Input: part model. Units: mm. Frame: model coordinates. A direction names the side the tool comes from. Give positions to 0.01 mm unless a question says otherwise; leave off trailing zeros. Loops run counter-clockwise (first coordinate to the right, second up) from the corner with the lowest first, then second, coordinate; pieces in that order, holes last. Notation, with made-up numbers: M 71,64 L 117,64 A25 cw 117,96 Z; hole C -17.5,18.5 d6. An arc over 180 degrees is marked long. Use CSV: the item, a comma, the result in double quotes. Start each with the question number.
from build123d import *

# Parameters (mm, degrees)
F1_DEPTH = 12.5
F2_R     = 6
F3_DEPTH = 20.001
F4_R     = 5
F5_R     = 12
F6_W     = 12
F6_H     = 90
F7_DEPTH = 20.001
F8_R     = 5.99999


# Not quite as in the source:
# - a fillet or chamfer is up to 0.001 mm smaller than in the source, because OpenCascade refuses the exact size


with BuildPart() as f1:
    # F0 (on Right) → F1 (new body, symmetric)
    with BuildSketch(Plane.YZ):
        Polygon((-6.25, 170), (-10, 170), (-10, -10), (10, -10), (10, 170), (6.25, 170), (6.25, 20), (-6.25, 20), align=None)
    extrude(amount=F1_DEPTH, both=True)

    # F2 (on face) → F3 (cut, through all)
    with BuildSketch(Plane.XZ.offset(10)):
        Circle(F2_R)
    extrude(amount=-F3_DEPTH, mode=Mode.SUBTRACT)

    # F4
    f4_edges = [f1.edges().sort_by_distance(p)[0] for p in [
        (12.5, 0, -10),
        (-12.5, 0, -10),
    ]]
    fillet(f4_edges, radius=F4_R)

    # F5
    f5_edges = [f1.edges().sort_by_distance(p)[0] for p in [
        (12.5, 0, 20),
        (-12.5, 0, 20),
    ]]
    fillet(f5_edges, radius=F5_R)

    # F6 (on face) → F7 (cut, through all)
    with BuildSketch(Plane.XZ.offset(10)):
        with Locations((0, 120)):
            Rectangle(F6_W, F6_H)
    extrude(amount=-F7_DEPTH, mode=Mode.SUBTRACT)

    # F8 (radius 6 in the source; OpenCascade refuses exactly that, so slightly less here)
    f8_edges = [f1.edges().sort_by_distance(p)[0] for p in [
        (-6, -8.125, 165),
        (6, -8.125, 165),
        (6, -8.125, 75),
        (-6, -8.125, 75),
        (-6, 8.125, 75),
        (6, 8.125, 75),
        (6, 8.125, 165),
        (-6, 8.125, 165),
    ]]
    fillet(f8_edges, radius=F8_R)


solid = f1.part
Item 1: Mould query, pull axis Y, two halves, no side actions, for faces 4 (the cylindrical face through (-4.196, 8.151, 76.711)), 5 (the flat face through (0, 10, 59)), 6 (the cylindrical face through (8.89, -0.09, 16.58)). Classes: +Y half, -Y half, draft (parallel to the pull), parting line (faces both ways), or undercut.
Item 2: Section A-A (z = 154.5). Output: boundary loops of the cut face in (x, y).
Item 3: Section B-B (z = 23.5). Output: boundary loops of the cut face in (x, y).
Item 4: Material intervals for line 1 (Y direction, x = 10, z = 45); line 2 (Z direction, x = 0, y = -3.5); line 3 (X direction, y = 2.25, z = 3), sorted ascending.
Item 5: Section D-D (z = 0). Output: boundary loops of the cut face in (x, y), then the cut area to 3 significant figures.
Item 6: First-contact query: pin 1 Ø9.5 at (x, z) = (0, 0) entering from +Y; pin 2 Ø3 at (x, y) = (9.5, 2) entering from +Z; pin 3 Ø0.8 at (x, y) = (0, -0.5) entering from +Z. Flat tips, straight axial feed; report the tip coordinate or a pass-through.
Item 7: Set-up query: faces 1 (the cylindrical face through (4.289, -8.099, 76.804)), 2 (the cylindrical face through (-9.08, -0.09, 16.39)), 3 (the cylindrical face through (11.07, 0.14, -8.5)). Return all of +Z, -Z, +X, -X, +Y, -Y with unobstructed straight access to the full face (end or side cutting, diameter ignored); none if empty.
Item 8: Section C-C (y = 3). Output: boundary loops of the cut face in (x, z), then the cut area to 3 significant figures.
Recorded:
1,face 4,"draft"
1,face 5,"+Y half"
1,face 6,"undercut"
2,outline,"M -12.5,-10 L -6,-10 L -6,-6.25 L -12.5,-6.25 Z; M -12.5,6.25 L -6,6.25 L -6,10 L -12.5,10 Z; M 6,-10 L 12.5,-10 L 12.5,-6.25 L 6,-6.25 Z; M 6,6.25 L 12.5,6.25 L 12.5,10 L 6,10 Z"
3,outline,"M -12.5,-10 L 12.5,-10 L 12.5,-6.25 L -12.5,-6.25 Z; M -12.5,6.25 L 12.5,6.25 L 12.5,10 L -12.5,10 Z"
4,line 1,"-10 to -6.25, 6.25 to 10"
4,line 2,"-10 to -6, 6 to 20"
4,line 3,"-12.5 to -5.2, 5.2 to 12.5"
5,outline,"M -12.5,-10 L -6,-10 L -6,10 L -12.5,10 Z; M 6,-10 L 12.5,-10 L 12.5,10 L 6,10 Z"
5,area,"260 mm²"
6,pin 1,"through"
6,pin 2,"z = 17.37"
6,pin 3,"z = 20"
7,face 1,"+Y, -Y"
7,face 2,"+Z, -X"
7,face 3,"-Z, +X, +Y, -Y"
8,outline,"M -12.5,-5 A5 ccw -7.5,-10 L 7.5,-10 A5 ccw 12.5,-5 L 12.5,8 A12 ccw 0.5,20 L -0.5,20 A12 ccw -12.5,8 Z; hole C 0,0 d12"
8,area,"564 mm²"
